from build123d import *

# Parameters (mm, degrees)
SKETCH1_W           = 300
SKETCH1_H           = 186
BOSS_EXTRUDE1_DEPTH = 6
FILLET1_R           = 94
CUT_EXTRUDE1_DEPTH  = 10
SKETCH3_W           = 70
SKETCH3_H           = 6
SKETCH3_W_2         = 6
SKETCH3_H_2         = 30
SKETCH3_W_3         = 122
SKETCH3_H_3         = 35
SKETCH3_W_4         = 30
SKETCH3_H_4         = 15
SKETCH3_W_5         = 132
CUT_EXTRUDE2_DEPTH  = 6
SKETCH4_R           = 0.9
CUT_EXTRUDE3_DEPTH  = 6


with BuildPart() as part:
    # Sketch1 → Boss-Extrude1 (new body)
    with BuildSketch(Plane.XY):
        Rectangle(SKETCH1_W, SKETCH1_H)
    extrude(amount=BOSS_EXTRUDE1_DEPTH)

    # Fillet1
    fillet1_edges = [part.edges().sort_by_distance(p)[0] for p in [
        (-150, 93, 3),
    ]]
    fillet(fillet1_edges, radius=FILLET1_R)

    # Sketch2 → Cut-Extrude1 (cut)
    with BuildSketch(Plane(origin=(0, 0, 0), x_dir=(-1, 0, 0), z_dir=(0, 0, -1))):
        with BuildLine():
            Line((110, -81), (30, -81))
            ThreePointArc((30, -81), (15.857864376, -75.142135624), (10, -61))
            Line((10, -61), (10, -41))
            ThreePointArc((10, -41), (15.857864376, -26.857864376), (30, -21))
            Line((30, -21), (110, -21))
            ThreePointArc((110, -21), (124.142135624, -26.857864376), (130, -41))
            Line((130, -41), (130, -61))
            ThreePointArc((130, -61), (124.142135624, -75.142135624), (110, -81))
        make_face()
    extrude(amount=-CUT_EXTRUDE1_DEPTH, mode=Mode.SUBTRACT)

    # Sketch3 → Cut-Extrude2 (cut)
    with BuildSketch(Plane.XY.offset(6)):
        with Locations((-75, -4)):
            Rectangle(SKETCH3_W, SKETCH3_H)
        with Locations((-147, -47)):
            Rectangle(SKETCH3_W_2, SKETCH3_H_2)
        with Locations((-74, -90)):
            Rectangle(SKETCH3_W_3, SKETCH3_H)
        with Locations((147, 45.5)):
            Rectangle(SKETCH3_W_2, SKETCH3_H_3)
        with Locations((147, -45.5)):
            Rectangle(SKETCH3_W_2, SKETCH3_H_3)
        with Locations((75, -4)):
            Rectangle(SKETCH3_W, SKETCH3_H)
        with Locations((0, -4)):
            Rectangle(SKETCH3_W_4, SKETCH3_H)
        with Locations((0, -29.5)):
            Rectangle(SKETCH3_W_2, SKETCH3_H_4)
        with Locations((0, -64.5)):
            Rectangle(SKETCH3_W_2, SKETCH3_H_4)
        with Locations((69, -90)):
            Rectangle(SKETCH3_W_5, SKETCH3_H)
    extrude(amount=-CUT_EXTRUDE2_DEPTH, mode=Mode.SUBTRACT)

    # Sketch4 → Cut-Extrude3 (cut)
    with BuildSketch(Plane(origin=(0, 0, 0), x_dir=(-1, 0, 0), z_dir=(0, 0, -1))):
        with Locations((130, -75)):
            Circle(SKETCH4_R)
        with Locations((130, -25)):
            Circle(SKETCH4_R)
        with Locations((10, -75)):
            Circle(SKETCH4_R)
        with Locations((10, -25)):
            Circle(SKETCH4_R)
    extrude(amount=-CUT_EXTRUDE3_DEPTH, mode=Mode.SUBTRACT)


solid = part.part
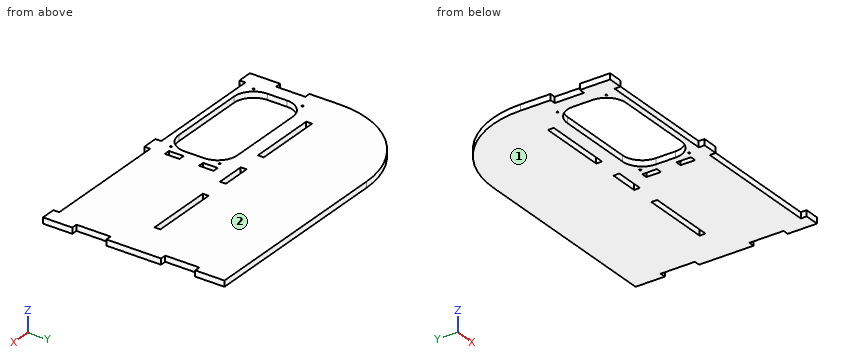
Could you check a few things on this model? Use its own coordinates, in mm. Face numbers are marked on the shaded views. Round coordinates to 2 decimals unless told otherwise and drop trailing zeros. Order: outer loops, then holes, each group sorted by start corner. A loop starts at its lowest first (then second) coordinate and runs counter-clockwise, first axis right, second up.
Q1. Thinking about a two-plate mould opening in Z: for the marked faces 1 and 2, which applies, released by +Z, released by -Z, zero draft, split by the parting line, or undercut?
Geometry says:
face 1: released by -Z
face 2: released by +Z
Q2. Imagine slicing it at A-A, the plane z = 2.5. State how many separate pieces and enclosed holes the cut face has, then the cut area to 3 significant figures.
Geometry says:
separate pieces: 1
enclosed holes: 10
area: 43,700 mm2
Q3. Imagine slicing it at C-C, the plane y = 75.5. List the corners of the cut face in (x, z) for me, then the cut area to 3 significant figures.
Geometry says:
outline: (-110.62, 0) - (150, 0) - (150, 6) - (-110.62, 6) - close
area: 1,560 mm2
Q4. Please list where these lines run through material, in increasing order: probe 1 along X at (y, z) = (-1.5, 3.6); probe 2 along Y at (x, z) = (-43, 2.55); probe 3 along X at (y, z) = (-58, 5.3).
Geometry says:
probe 1: x = -150 to -110, -40 to -15, 15 to 40, 110 to 150
probe 2: y = -87 to -81, -21 to -7, -1 to 93
probe 3: x = -144 to -130, -10 to -3, 3 to 144
Q5. Imagine slicing it at B-B, the plane x = 18.5. List the corners of the cut face in (y, z) for me.
Geometry says:
outline: (-87, 0) - (93, 0) - (93, 6) - (-87, 6) - close
Q6. I'm going to push a flat-ended pin straight in: P1, Ø3, axis at y = -37.5, z = 3, coming from the -X side. Where does the tip first touch, or does it pass through?
Geometry says:
P1: stops at x = -144
